from build123d import *

# Parameters (mm, degrees)
F0_W      = 40
F0_H      = 70
F1_DEPTH  = 50
F2_W      = 40
F2_H      = 70
F3_DEPTH  = 40
F4_W      = 30
F4_H      = 33
F5_DEPTH  = 70
F6_W      = 30
F6_H      = 43
F7_DEPTH  = 70
F8_R      = 2
F9_R      = 1.875
F10_DEPTH = 15


with BuildPart() as f1:
    # F0 (on Top) → F1 (new body)
    with BuildSketch(Plane.XY):
        with Locations((0, 35)):
            Rectangle(F0_W, F0_H)
    extrude(amount=F1_DEPTH)

    # F2 (on Top) → F3 (join)
    with BuildSketch(Plane.XY):
        with Locations((0, -35)):
            Rectangle(F2_W, F2_H)
    extrude(amount=F3_DEPTH)

    # F4 (on face) → F5 (cut)
    with BuildSketch(Plane.XZ.offset(70)):
        with Locations((0, 21.5)):
            Rectangle(F4_W, F4_H)
    extrude(amount=-F5_DEPTH, mode=Mode.SUBTRACT)

    # F6 (on face) → F7 (cut)
    with BuildSketch(Plane(origin=(0, 70, 0), x_dir=(-1, 0, 0), z_dir=(0, 1, 0))):
        with Locations((0, 26.5)):
            Rectangle(F6_W, F6_H)
    extrude(amount=-F7_DEPTH, mode=Mode.SUBTRACT)

    # F8
    f8_edges = [f1.edges().sort_by_distance(p)[0] for p in [
        (-15, 0, 5),
        (15, 0, 5),
        (15, -35, 38),
        (-15, -35, 38),
        (15, 35, 48),
        (-15, 35, 48),
    ]]
    fillet(f8_edges, radius=F8_R)

    # F9 (on face) → F10 (cut)
    with BuildSketch(Plane.XY.offset(50)):
        with Locations((5, 65)):
            Circle(F9_R)
        with Locations((5, 60)):
            Circle(F9_R)
        with Locations((5, 55)):
            Circle(F9_R)
        with Locations((5, 50)):
            Circle(F9_R)
        with Locations((5, 45)):
            Circle(F9_R)
        with Locations((5, 40)):
            Circle(F9_R)
        with Locations((5, 35)):
            Circle(F9_R)
        with Locations((5, 30)):
            Circle(F9_R)
        with Locations((5, 25)):
            Circle(F9_R)
        with Locations((5, 20)):
            Circle(F9_R)
        with Locations((5, 15)):
            Circle(F9_R)
        with Locations((5, 10)):
            Circle(F9_R)
        with Locations((5, 5)):
            Circle(F9_R)
        with Locations((5, -5)):
            Circle(F9_R)
        with Locations((5, -10)):
            Circle(F9_R)
        with Locations((5, -15)):
            Circle(F9_R)
        with Locations((5, -20)):
            Circle(F9_R)
        with Locations((5, -25)):
            Circle(F9_R)
        with Locations((5, -30)):
            Circle(F9_R)
        with Locations((5, -35)):
            Circle(F9_R)
        with Locations((5, -40)):
            Circle(F9_R)
        with Locations((5, -45)):
            Circle(F9_R)
        with Locations((5, -50)):
            Circle(F9_R)
        with Locations((5, -55)):
            Circle(F9_R)
        with Locations((5, -60)):
            Circle(F9_R)
        with Locations((5, -65)):
            Circle(F9_R)
        with Locations((-5, 65)):
            Circle(F9_R)
        with Locations((-5, 60)):
            Circle(F9_R)
        with Locations((-5, 55)):
            Circle(F9_R)
        with Locations((-5, 50)):
            Circle(F9_R)
        with Locations((-5, 45)):
            Circle(F9_R)
        with Locations((-5, 40)):
            Circle(F9_R)
        with Locations((-5, 35)):
            Circle(F9_R)
        with Locations((-5, 30)):
            Circle(F9_R)
        with Locations((-5, 25)):
            Circle(F9_R)
        with Locations((-5, 20)):
            Circle(F9_R)
        with Locations((-5, 15)):
            Circle(F9_R)
        with Locations((-5, 10)):
            Circle(F9_R)
        with Locations((-5, 5)):
            Circle(F9_R)
        with Locations((-5, -5)):
            Circle(F9_R)
        with Locations((-5, -10)):
            Circle(F9_R)
        with Locations((-5, -15)):
            Circle(F9_R)
        with Locations((-5, -20)):
            Circle(F9_R)
        with Locations((-5, -25)):
            Circle(F9_R)
        with Locations((-5, -30)):
            Circle(F9_R)
        with Locations((-5, -35)):
            Circle(F9_R)
        with Locations((-5, -40)):
            Circle(F9_R)
        with Locations((-5, -45)):
            Circle(F9_R)
        with Locations((-5, -50)):
            Circle(F9_R)
        with Locations((-5, -55)):
            Circle(F9_R)
        with Locations((-5, -60)):
            Circle(F9_R)
        with Locations((-5, -65)):
            Circle(F9_R)
    extrude(amount=-F10_DEPTH, mode=Mode.SUBTRACT)


solid = f1.part
Geometry check sheet. Reference: the model listing, model coordinates, mm. A direction names the side the tool comes from. Give positions to 0.01 mm unless a question says otherwise; leave off trailing zeros. Write each loop counter-clockwise with the first axis right and the second up, starting at its lowest first coordinate (ties: lowest second). Pieces come first, ordered by that corner, then holes.
1) Release check for a two-part mould opening along Y. For faces 1 (the face through (-5.24, 51.86, 49.01)), 2 (the face through (-0.3, 0, 48.3)), 3 (the face through (15, -1, 26)) record: released by +Y, released by -Y, zero draft, split by the parting line, or undercut.
Values follow:
face 1: undercut
face 2: released by -Y
face 3: zero draft
2) Cross-section at A-A (y = 25). Record the boundary of the cut face in (x, z) (3 decimals).
Values follow:
outline: (-20, 0) - (20, 0) - (20, 50) - (6.875, 50) - (6.875, 48) - (13, 48) arc R2 cw to (15, 46) - (15, 7) arc R2 cw to (13, 5) - (-13, 5) arc R2 cw to (-15, 7) - (-15, 46) arc R2 cw to (-13, 48) - (-6.875, 48) - (-6.875, 50) - (-20, 50) - close; (-3.125, 48) - (3.125, 48) - (3.125, 50) - (-3.125, 50) - close
3) Set-up check for faces 4 (the face through (-5.24, -48.14, 39.01)), 5 (the face through (0, 0, 39)), 6 (the face through (0, 1, 0)): record each of +Z, -Z, +X, -X, +Y, -Y from which the full face is reachable in a straight line by a thin tool's end or side.
Values follow:
face 4: +Z
face 5: +Y
face 6: -Z, +X, -X, +Y, -Y
4) Cross-section at C-C (z = 8.5). Record the boundary of the cut face in (x, y).
Values follow:
outline: (-20, -70) - (-15, -70) - (-15, 70) - (-20, 70) - close; (15, -70) - (20, -70) - (20, 70) - (15, 70) - close
5) Thickness scan on line 1 (X direction, y = 0, z = 23); line 2 (Z direction, x = -7.5, y = -2.5); line 3 (Z direction, x = 6, y = 35). Record the ranges inside material, lowest first.
Values follow:
line 1: x = -20 to -15, 15 to 20
line 2: z = 0 to 5, 38 to 40
line 3: z = 0 to 5
6) Cross-section at B-B (x = -1.5). Record the boundary of the cut face in (y, z).
Values follow:
outline: (-70, 0) - (70, 0) - (70, 5) - (-70, 5) - close; (-70, 38) - (0, 38) - (0, 40) - (-70, 40) - close; (0, 48) - (70, 48) - (70, 50) - (0, 50) - close
7) Cross-section at D-D (x = -17). Record the boundary of the cut face in (y, z), plus the area to 3 significant figures.
Values follow:
outline: (-70, 0) - (70, 0) - (70, 50) - (0, 50) - (0, 40) - (-70, 40) - close
area: 6,300 mm2
8) Go/stop test with flat-tipped pins: pin 1 Ø6 at (x, y) = (5, -10) entering from +Z; pin 2 Ø2 at (x, y) = (5, -30) entering from +Z. Record where each tip stops, or that it passes through.
Values follow:
pin 1: stops at z = 40
pin 2: stops at z = 5
